from build123d import *

# Parameters (mm, degrees)
SKETCH1_W           = 55.675357375
SKETCH1_H           = 69.594196719
BOSS_EXTRUDE1_DEPTH = 6


with BuildPart() as part:
    # Sketch1 → Boss-Extrude1 (new body)
    with BuildSketch(Plane(origin=(0, 0, 0), x_dir=(0, 0, -1), z_dir=(1, 0, 0))):
        Polygon((36, -45), (27.5, -45), (27.5, -51), (12.5, -51), (12.5, -45), (-12.5, -45), (-12.5, -51), (-27.5, -51), (-27.5, -45), (-36, -45), (-36, -27.5), (-42, -27.5), (-42, -12.5), (-36, -12.5), (-36, 12.5), (-42, 12.5), (-42, 27.5), (-36, 27.5), (-36, 45), (-27.5, 45), (-27.5, 51), (-12.5, 51), (-12.5, 45), (12.5, 45), (12.5, 51), (27.5, 51), (27.5, 45), (36, 45), (36, 27.5), (42, 27.5), (42, 12.5), (36, 12.5), (36, -12.5), (42, -12.5), (42, -27.5), (36, -27.5), align=None)
        with Locations((0.337678688, -0.42209836)):
            Rectangle(SKETCH1_W, SKETCH1_H, mode=Mode.SUBTRACT)
    extrude(amount=BOSS_EXTRUDE1_DEPTH)


solid = part.part
Geometry: final body of the model. Coordinates: model frame, mm. A direction names the side the tool comes from. Coordinates: 2 decimals unless noted, no trailing zeros. Order: outer loops, then holes, each group sorted by start corner. A loop starts at its lowest first (then second) coordinate and runs counter-clockwise, first axis right, second up. Notation, with made-up numbers: (53, 68.5) - (66, 68.5) arc R26 cw to (66, 96.5) - close; hole circle Ø5 at (69.25, 53). An arc over 180 degrees is marked (long way). Use one line per item in the form item = value.
1) Section C-C (y = 42.5). Return loops of the section in (x, z), then the cut area to 3 significant figures.
Solutions:
outline = (0, -36) - (6, -36) - (6, 36) - (0, 36) - close
area = 432 mm^2
2) Set-up query: faces 4 (the face through (3, 45, -32)), 5 (the face through (3, -35.219, 0)), 6 (the face through (3, -27.5, 39)), 7 (the face through (3, 45, 32)). Return all of +Z, -Z, +X, -X, +Y, -Y with unobstructed straight access to the full face (end or side cutting, diameter ignored); none if empty.
Solutions:
face_4 = -Z, +X, -X, +Y
face_5 = +X, -X
face_6 = +Z, +X, -X, -Y
face_7 = +Z, +X, -X, +Y
3) Section A-A (y = -34). Return loops of the section in (x, z).
Solutions:
outline = (0, -36) - (6, -36) - (6, -28.18) - (0, -28.18) - close; (0, 27.5) - (6, 27.5) - (6, 36) - (0, 36) - close
4) Section B-B (z = -9). Return loops of the section in (x, y) (3 decimals), then the cut area to 3 significant figures.
Solutions:
outline = (0, -45) - (6, -45) - (6, -35.219) - (0, -35.219) - close; (0, 34.375) - (6, 34.375) - (6, 45) - (0, 45) - close
area = 122 mm^2
5) Mould query, pull axis Z, two halves, no side actions, for faces 1 (the face through (3, -51, 20)), 2 (the face through (3, 20, -42)), 3 (the face through (3, 45, 0)). Classes: +Z half, -Z half, draft (parallel to the pull), parting line (faces both ways), or undercut.
Solutions:
face_1 = draft
face_2 = -Z half
face_3 = undercut
6) Ray query, L1, parallel to Y at x = 4.8, z = -21.5 (3 decimals); L2, parallel to Y at x = 0.8, z = -36.5; L3, parallel to Z at x = 0.35, y = -15. Return the intervals inside material, ascending.
Solutions:
L1 = -51 to -35.219, 34.375 to 51
L2 = -27.5 to -12.5, 12.5 to 27.5
L3 = -42 to -28.18, 27.5 to 42
7) Pin query (flat end, axial travel): pin 1 (2 mm diameter, centred on x = 3, y = 2, fed in from -Z); pin 2 (1.8 mm diameter, centred on x = 3, y = 48.5, fed in from +Z); pin 3 (1.8 mm diameter, centred on x = 3.5, z = 40, fed in from +Y). Return the tip coordinate at first contact, or that it passes through.
Solutions:
pin_1 = -36
pin_2 = 27.5
pin_3 = 27.5
